For this review, take the finished solid that the model builds, in its own axes (mm). A direction names the side the tool comes from. Coordinates: 2 decimals unless noted, no trailing zeros. Write each loop counter-clockwise with the first axis right and the second up, starting at its lowest first coordinate (ties: lowest second). Pieces come first, ordered by that corner, then holes. Notation, with made-up numbers: (-36.75, 70) -> (13.25, 70) arc R29 cw to (13.25, 94) -> close; hole circle Ø4 at (6.5, 12.5). An arc over 180 degrees is marked (long way). One line per item, written item: value. Start each with the question number.
1) For probe 1 along X at (y, z) = (1.35, -1.25); probe 2 along Y at (x, z) = (3.5, -1.5), list the stretches that pass through material, from the lowest coordinate up. Write a range as from..to.
2) Add section D-D (z = -3). State the section outline as (x, y) points, and give its area (3 significant figures).
3) Mouldability with a two-part tool opening along Z and no side actions: class faces 1 (the flat face through (0, 5, 0)), 2 (the flat face through (-3.7, 1, 0)), 3 (the flat face through (0.67, 3.99, 0.69)) as released by +Z, released by -Z, zero draft, split by the parting line, or undercut.
4) Add section B-B (x = -0.25). State the section outline as (y, z) points.
5) Add section C-C (z = -1.25). State the section outline as (x, y) points, and give its area (3 significant figures).
6) For pin 1 Ø1 at (x, z) = (-1, 0.5) entering from +Y; pin 2 Ø1.5 at (x, z) = (-1, -0.5) entering from -Y; pin 3 Ø1.5 at (x, y) = (1, 1) entering from +Z, all flat-tipped, find the tip position at first contact; note any pin that passes through.
7) Machinability: for faces 4 (the cylindrical face through (-1.5, 2.44, -0.07)), 5 (the flat face through (0.69, 3.99, -0.67)), 6 (the cylindrical face through (-0.1, -0.25, 1.46)), 7 (the flat face through (-0.67, 3.99, -0.69)), which of the approach directions +Z, -Z, +X, -X, +Y, -Y give a long, thin tool a straight path to every point of the face, cutting with its end or side? Answer none if there is none.
from build123d import *

# Parameters (mm, degrees)
SZKIC2_W                    = 7.4
SZKIC2_H                    = 7.4
DODANIE_WYCI_GNI_CIE1_DEPTH = 1.9
DODANIE_WYCI_GNI_CIE2_START = -1.9
DODANIE_WYCI_GNI_CIE2_DEPTH = 5
DODANIE_WYCI_GNI_CIE3_START = -1.9
SZKIC4_R                    = 1.5
DODANIE_WYCI_GNI_CIE3_DEPTH = 3
SZKIC5_R                    = 0.45
DODANIE_WYCI_GNI_CIE4_DEPTH = 0.5
SZKIC6_W                    = 0.8
SZKIC6_H                    = 0.8
DODANIE_WYCI_GNI_CIE5_DEPTH = 0.2
ZAOKR_GLENIE1_R             = 1
SZKIC7_W                    = 1.2
SZKIC7_H                    = 0.9
DODANIE_WYCI_GNI_CIE6_DEPTH = 0.2


with BuildPart() as part:
    # Szkic2 → Dodanie-wyciągnięcie1 (new body)
    with BuildSketch(Plane(origin=(0, 0, 0), x_dir=(1, 0, 0), z_dir=(0, 1, 0))):
        Rectangle(SZKIC2_W, SZKIC2_H)
    extrude(amount=DODANIE_WYCI_GNI_CIE1_DEPTH)

    # Szkic3 → Dodanie-wyciągnięcie2 (add)
    with BuildSketch(Plane(origin=(0, 1.9, 0), x_dir=(1, 0, 0), z_dir=(0, 1, 0)).offset(DODANIE_WYCI_GNI_CIE2_START)):
        Polygon((0, -1.35764502), (1.35764502, 0), (0, 1.35764502), (-1.35764502, 0), align=None)
    extrude(amount=DODANIE_WYCI_GNI_CIE2_DEPTH)

    # Szkic4 → Dodanie-wyciągnięcie3 (add)
    with BuildSketch(Plane(origin=(0, 1.9, 0), x_dir=(1, 0, 0), z_dir=(0, 1, 0)).offset(DODANIE_WYCI_GNI_CIE3_START)):
        Circle(SZKIC4_R)
    extrude(amount=DODANIE_WYCI_GNI_CIE3_DEPTH)

    # Szkic5 → Dodanie-wyciągnięcie4 (add)
    with BuildSketch(Plane.XZ):
        with Locations((0, 1.9)):
            Circle(SZKIC5_R)
        with Locations((0, -1.9)):
            Circle(SZKIC5_R)
    extrude(amount=DODANIE_WYCI_GNI_CIE4_DEPTH)

    # Szkic6 → Dodanie-wyciągnięcie5 (add)
    with BuildSketch(Plane(origin=(3.7, 0, 0), x_dir=(0, 0, -1), z_dir=(1, 0, 0))):
        with Locations((-1.4, 0.4)):
            Rectangle(SZKIC6_W, SZKIC6_H)
        with Locations((0, 0.4)):
            Rectangle(SZKIC6_W, SZKIC6_H)
        with Locations((1.4, 0.4)):
            Rectangle(SZKIC6_W, SZKIC6_H)
    dodanie_wyci_gni_cie5 = extrude(amount=DODANIE_WYCI_GNI_CIE5_DEPTH)

    # Lustro1: Dodanie-wyciągnięcie5 across plane
    add(dodanie_wyci_gni_cie5.mirror(Plane(origin=(0, 0, 0), x_dir=(0, 0, 1), z_dir=(1, 0, 0))))

    # Zaokrąglenie1
    zaokr_glenie1_edges = [part.edges().sort_by_distance(p)[0] for p in [
        (3.7, 0.95, 3.7),
        (-3.7, 0.95, 3.7),
        (-3.7, 0.95, -3.7),
        (3.7, 0.95, -3.7),
    ]]
    fillet(zaokr_glenie1_edges, radius=ZAOKR_GLENIE1_R)

    # Szkic7 → Dodanie-wyciągnięcie6 (add)
    with BuildSketch(Plane.XZ):
        with Locations((0, 3.7)):
            Rectangle(SZKIC7_W, SZKIC7_H)
        with Locations((0, -3.7)):
            Rectangle(SZKIC7_W, SZKIC7_H)
    extrude(amount=-DODANIE_WYCI_GNI_CIE6_DEPTH)


solid = part.part
Numbers:
1. probe 1: -3.7..3.7
1. probe 2: 0..1.9
2. outline: (-3.65, 0) -> (3.65, 0) -> (3.65, 1.9) -> (-3.65, 1.9) -> close
2. area: 13.9 mm²
3. face 1: zero draft
3. face 2: undercut
3. face 3: released by +Z
4. outline: (-0.5, -2.27) -> (0, -2.27) -> (0, -4.15) -> (0.2, -4.15) -> (0.2, -3.7) -> (1.9, -3.7) -> (1.9, -1.48) -> (3, -1.48) -> (3, -1.11) -> (5, -1.11) -> (5, 1.11) -> (3, 1.11) -> (3, 1.48) -> (1.9, 1.48) -> (1.9, 3.7) -> (0.2, 3.7) -> (0.2, 4.15) -> (0, 4.15) -> (0, 2.27) -> (-0.5, 2.27) -> (-0.5, 1.53) -> (0, 1.53) -> (0, -1.53) -> (-0.5, -1.53) -> close
5. outline: (-3.9, 0) -> (3.9, 0) -> (3.9, 0.8) -> (3.7, 0.8) -> (3.7, 1.9) -> (0.83, 1.9) -> (0.83, 3) -> (0.11, 3) -> (0.11, 5) -> (-0.11, 5) -> (-0.11, 3) -> (-0.83, 3) -> (-0.83, 1.9) -> (-3.7, 1.9) -> (-3.7, 0.8) -> (-3.9, 0.8) -> close
5. area: 16.6 mm²
6. pin 1: y = 5
6. pin 2: y = 0
6. pin 3: z = 3.7
7. face 4: +Y
7. face 5: -Z, +X, +Y
7. face 6: -Y
7. face 7: -Z, -X, +Y
